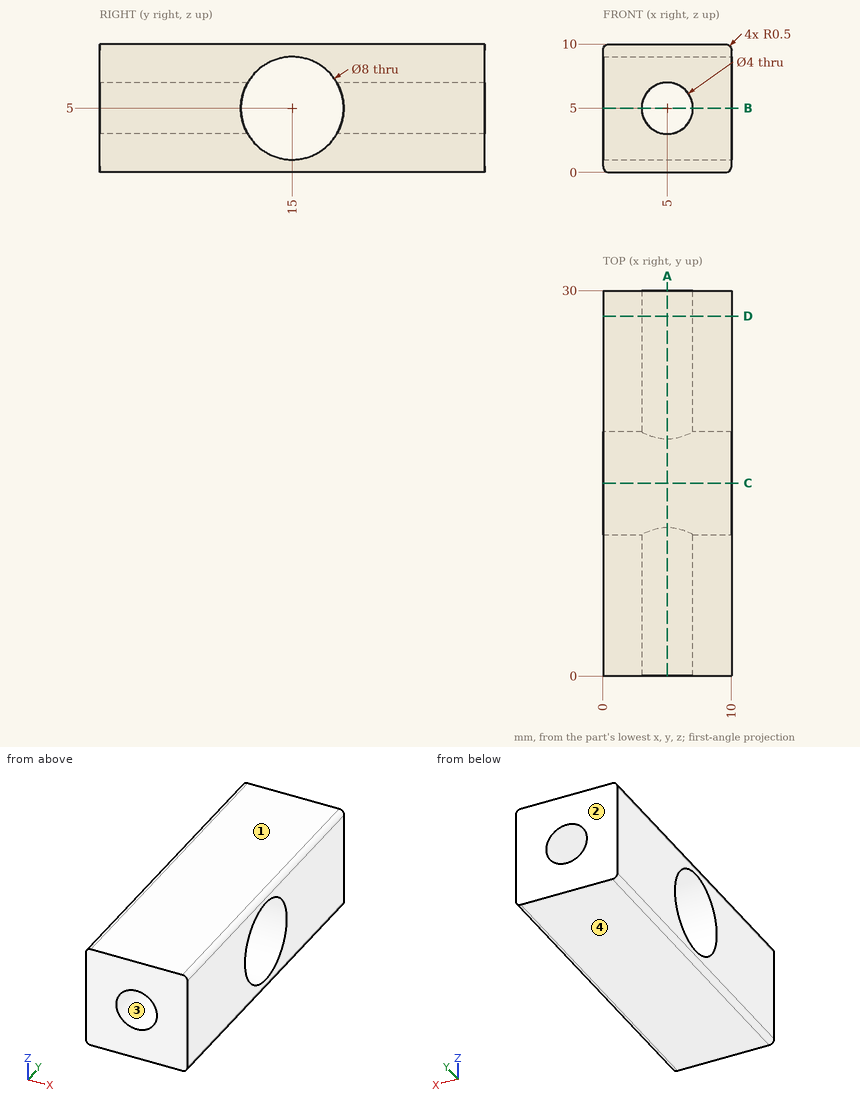
Answer from the drawing. Dimensions are ordinates in mm from the lowest x, y and z of the part. Coordinates: 2 decimals unless noted, no trailing zeros. Order: outer loops, then holes, each group sorted by start corner. A loop starts at its lowest first (then second) coordinate and runs counter-clockwise, first axis right, second up. Notation, with made-up numbers: (26.25, -15.5) - (78.25, -15.5) arc R21 ccw to (78.25, 16.5) - close; hole circle Ø9 at (18, 48). An arc over 180 degrees is marked (long way). Answer as a JSON object with one key per item and string values. Group by question number.
Item 1: Section D-D (y = 28) is taken. Give the vertices of the cut face in (x, z).
Item 2: The mould has two halves that part along Z. Classify the marked faces 1, 2, 3 and 4: +Z half, -Z half, draft (parallel to the pull), parting line (faces both ways), or undercut.
Item 3: Section A-A (x = 5) is taken. Give the vertices of the cut face in (y, z).
Item 4: Consider probe 1 along Z at (x, y) = (5, 9); probe 2 along Z at (x, y) = (7.75, 15). Determine where each line is inside the solid, lowest interval first. Write a range as from..to.
Item 5: Section B-B (z = 5) is taken. Give the vertices of the cut face in (x, y), plus the area to 3 significant figures.
Item 6: Section C-C (y = 15) is taken. Give the vertices of the cut face in (x, z).
Results are:
{
 "1": {"outline": "(0, 0.5) arc R0.5 ccw to (0.5, 0) - (9.5, 0) arc R0.5 ccw to (10, 0.5) - (10, 9.5) arc R0.5 ccw to (9.5, 10) - (0.5, 10) arc R0.5 ccw to (0, 9.5) - close; hole circle Ø4 at (5, 5)"},
 "2": {"face 1": "+Z half", "face 2": "draft", "face 3": "undercut", "face 4": "-Z half"},
 "3": {"outline": "(0, 0) - (30, 0) - (30, 3) - (18.46, 3) arc R4 cw to (11.54, 3) - (0, 3) - close; (0, 7) - (11.54, 7) arc R4 cw to (18.46, 7) - (30, 7) - (30, 10) - (0, 10) - close"},
 "4": {"probe 1": "z = 0..3, 7..10", "probe 2": "z = 0..1, 9..10"},
 "5": {"outline": "(0, 0) - (3, 0) - (3, 11) - (0, 11) - close; (0, 19) - (3, 19) - (3, 30) - (0, 30) - close; (7, 0) - (10, 0) - (10, 11) - (7, 11) - close; (7, 19) - (10, 19) - (10, 30) - (7, 30) - close", "area": "132 mm^2"},
 "6": {"outline": "(0, 0.5) arc R0.5 ccw to (0.5, 0) - (9.5, 0) arc R0.5 ccw to (10, 0.5) - (10, 1) - (0, 1) - close; (0, 9) - (10, 9) - (10, 9.5) arc R0.5 ccw to (9.5, 10) - (0.5, 10) arc R0.5 ccw to (0, 9.5) - close"}
}
